from build123d import *

# Parameters (mm, degrees)
BOSS_EXTRUDE1_DEPTH = 65.024
SKETCH8_R           = 1.524
BOSS_EXTRUDE4_DEPTH = 7.62
SKETCH9_R           = 2.794
BOSS_EXTRUDE5_DEPTH = 3.81


with BuildPart() as part:
    # Sketch2 → Boss-Extrude1 (new body)
    with BuildSketch(Plane(origin=(0, 273.277204506, 0), x_dir=(1, 0, 0), z_dir=(0, 1, 0))):
        with BuildLine():
            Line((-29.45165626, 3.139900531), (-29.45165626, 3.311685007))
            Line((-29.45165626, 3.311685007), (-63.74165626, 3.311685007))
            Line((-63.74165626, 3.311685007), (-63.74165626, 4.581685007))
            Line((-63.74165626, 4.581685007), (10.93434374, 4.581685007))
            Line((10.93434374, 4.581685007), (10.93434374, 3.311685007))
            Line((10.93434374, 3.311685007), (-23.35565626, 3.311685007))
            Line((-23.35565626, 3.311685007), (-23.35565626, 3.139900531))
            Line((-23.35565626, 3.139900531), (-23.35565626, 0.345900531))
            Line((-23.35565626, 0.345900531), (-19.572733097, 0.345900531))
            ThreePointArc((-19.572733097, 0.345900531), (-19.220734995, 0.110702919), (-19.303325413, -0.304507152))
            Line((-19.303325413, -0.304507152), (-23.190363831, -4.19154557))
            ThreePointArc((-23.190363831, -4.19154557), (-23.931995607, -4.68708808), (-24.806809933, -4.861099469))
            Line((-24.806809933, -4.861099469), (-28.000502588, -4.861099469))
            ThreePointArc((-28.000502588, -4.861099469), (-28.875316914, -4.68708808), (-29.616948689, -4.19154557))
            Line((-29.616948689, -4.19154557), (-33.503987108, -0.304507152))
            ThreePointArc((-33.503987108, -0.304507152), (-33.586577526, 0.110702919), (-33.234579424, 0.345900531))
            Line((-33.234579424, 0.345900531), (-29.45165626, 0.345900531))
            Line((-29.45165626, 0.345900531), (-29.45165626, 3.139900531))
        make_face()
    extrude(amount=-BOSS_EXTRUDE1_DEPTH)

    # Sketch8 → Boss-Extrude4 (add)
    with BuildSketch(Plane(origin=(0, 0, -4.581685007), x_dir=(-1, 0, 0), z_dir=(0, 0, -1))):
        with Locations((7.624251866, 262.75164523)):
            Circle(SKETCH8_R)
        with Locations((58.424251866, 247.51164523)):
            Circle(SKETCH8_R)
        with Locations((58.424251866, 219.57164523)):
            Circle(SKETCH8_R)
        with Locations((6.354251866, 214.49164523)):
            Circle(SKETCH8_R)
    extrude(amount=BOSS_EXTRUDE4_DEPTH)

    # Sketch9 → Boss-Extrude5 (add)
    with BuildSketch(Plane(origin=(0, 0, -4.581685007), x_dir=(-1, 0, 0), z_dir=(0, 0, -1))):
        with Locations((7.624251866, 262.75164523)):
            Circle(SKETCH9_R)
        with Locations((58.424251866, 247.51164523)):
            Circle(SKETCH9_R)
        with Locations((6.354251866, 214.49164523)):
            Circle(SKETCH9_R)
        with Locations((58.424251866, 219.57164523)):
            Circle(SKETCH9_R)
    extrude(amount=BOSS_EXTRUDE5_DEPTH)


solid = part.part
Could you check a few things on this model? Use its own coordinates, in mm. A direction names the side the tool comes from. Round coordinates to 2 decimals unless told otherwise and drop trailing zeros. Order: outer loops, then holes, each group sorted by start corner. A loop starts at its lowest first (then second) coordinate and runs counter-clockwise, first axis right, second up.
Q1. Which directions (+Z, -Z, +X, -X, +Y, -Y) give clear straight access to the entire face, cutting with the end or side of a thin tool? Please do faces 4 (the face through (-6, 215, -12.202)), 5 (the face through (-29.452, 241, -2)), 6 (the face through (-26, 241, 4.861)), 7 (the face through (-23.356, 241, -2)), 8 (the face through (-7.426, 264.263, -10.27)).
Geometry says:
face 4: -Z, +X, -X, +Y, -Y
face 5: -X, +Y, -Y
face 6: +Z, +X, -X, +Y, -Y
face 7: +X, +Y, -Y
face 8: -Z
Q2. Please list where these lines run through material, in increasing order: probe 1 along X at (y, z) = (245, -2.75); probe 2 along Z at (x, y) = (-6, 269.5); probe 3 along Z at (x, y) = (-20.5, 269.5).
Geometry says:
probe 1: x = -29.45 to -23.36
probe 2: z = -4.58 to -3.31
probe 3: z = -4.58 to -3.31, -0.35 to 1.5
Q3. Thinking about a two-plate mould opening in Y: for faces 1 (the face through (-8.8, 261.5, -8.392)), 2 (the face through (-26, 273.277, -2)), 3 (the face through (-6, 241, -3.312)), which applies, released by +Y, released by -Y, zero draft, split by the parting line, or undercut?
Geometry says:
face 1: undercut
face 2: released by +Y
face 3: zero draft
Q4. Imagine slicing it at A-A, the plane y = 233. List the corners of the cut face in (x, z) for me.
Geometry says:
outline: (-63.74, -4.58) - (10.93, -4.58) - (10.93, -3.31) - (-23.36, -3.31) - (-23.36, -0.35) - (-19.57, -0.35) arc R0.38 ccw to (-19.3, 0.3) - (-23.19, 4.19) arc R2.29 ccw to (-24.81, 4.86) - (-28, 4.86) arc R2.29 ccw to (-29.62, 4.19) - (-33.5, 0.3) arc R0.38 ccw to (-33.23, -0.35) - (-29.45, -0.35) - (-29.45, -3.31) - (-63.74, -3.31) - close
Q5. Imagine slicing it at D-D, the plane z = -7.5. List the corners of the cut face in (x, y) for me.
Geometry says:
outline: circle Ø5.59 at (-58.42, 219.57); circle Ø5.59 at (-58.42, 247.51); circle Ø5.59 at (-7.62, 262.75); circle Ø5.59 at (-6.35, 214.49)
Q6. Imagine slicing it at B-B, the plane z = -1.25. List the corners of the cut face in (x, y) for me.
Geometry says:
outline: (-29.45, 208.25) - (-23.36, 208.25) - (-23.36, 273.28) - (-29.45, 273.28) - close
Q7. I'm going to push flat-ended pins straight in: P1, Ø0.9, axis at y = 249.5, z = -2.5, coming from the -X side; P2, Ø10.5, axis at x = -44.5, y = 235.5, coming from the +Z side; P3, Ø4, axis at x = -32, y = 249, coming from the -Z side; P4, Ø3.5, axis at y = 250, z = -2.5, coming from the +X side. Where does each tip first touch, or does it pass through?
Geometry says:
P1: stops at x = -29.45
P2: stops at z = -3.31
P3: stops at z = -4.58
P4: stops at x = 10.93
Q8. Imagine slicing it at C-C, the plane x = -37.5. List the corners of the cut face in (y, z) for me, then the cut area to 3 significant figures.
Geometry says:
outline: (208.25, -4.58) - (273.28, -4.58) - (273.28, -3.31) - (208.25, -3.31) - close
area: 82.6 mm2
